Input: part model. Units: mm. Frame: model coordinates. Give positions to 0.01 mm unless a question says otherwise; leave off trailing zeros. Loops run counter-clockwise (first coordinate to the right, second up) from the corner with the lowest first, then second, coordinate; pieces in that order, holes last. Notation, with made-up numbers: (73.25, 84) -> (79.25, 84) arc R14 ccw to (79.25, 94) -> close; hole circle Ø1 at (39, 23.5). An arc over 180 degrees is marked (long way). Answer as a JSON object with one key per item and string values.
Autodesk Inventor part; units mm, degrees
ref_plane "YZ Plane" through (0, 0, 0) normal (1, 0, 0) x (0, 1, 0)
ref_plane "XZ Plane" through (0, 0, 0) normal (0, 1, 0) x (-1, 0, 0)
ref_plane "XY Plane" through (0, 0, 0) normal (0, 0, 1) x (1, 0, 0)
sketch "Sketch1" plane through (0, 0, 0) normal (0, 1, 0) x (-1, 0, 0)
  line L0 (1.9345, 2.6954) -> (3.3015, -0.3277)
  line L1 (3.3015, -0.3277) -> (1.367, -3.0231)
  line L2 (1.367, -3.0231) -> (-1.9345, -2.6954)
  line L3 (-1.9345, -2.6954) -> (-3.3015, 0.3277)
  line L4 (-3.3015, 0.3277) -> (-1.367, 3.0231)
  line L5 (-1.367, 3.0231) -> (1.9345, 2.6954)
  point P0 (0, 0)
  point P1 (0, 0)
extrude "Extrusion1" add sketch "Sketch1" along normal blind 19.05
sketch "Sketch2" plane through (0, 19.05, 0) normal (0, 1, 0) x (1, 0, 0)
  point P0 (0, 0)
  point P1 (0, 0)
hole "Hole1" at (0, 19.05, 0) direction (0, -1, 0) diameter 2.4892 end through all
properties part number "standoff"
Q1. Section C-C, the plane y = 2.5. Return the cut outline in (x, z).
Evaluation:
{"outline": "(-3.3, -0.33) -> (-1.37, -3.02) -> (1.93, -2.7) -> (3.3, 0.33) -> (1.37, 3.02) -> (-1.93, 2.7) -> close; hole circle Ø2.49 at (0, 0)"}
Q2. Ray query, line 1 along Z through (x, y) = (0, 5.25); line 2 along Z through (x, y) = (0.5, 10); line 3 along X through (y, z) = (5.25, 0). Return the intervals inside material, ascending.
Evaluation:
{"line 1": "z = -2.89 to -1.24, 1.24 to 2.89", "line 2": "z = -2.84 to -1.14, 1.14 to 2.94", "line 3": "x = -3.15 to -1.24, 1.24 to 3.15"}
Q3. Draft query along X for faces 1 (the cylindrical face through (-0.37, 9.39, 1.19)), 2 (the flat face through (0, 19.05, 1.4)), 3 (the flat face through (0.26, 9.39, -2.86)). Return one class per face: +X half, -X half, draft (parallel to the pull), parting line (faces both ways), or undercut.
Evaluation:
{"face 1": "undercut", "face 2": "draft", "face 3": "+X half"}
Q4. Section D-D, the plane z = -1.5. Return the cut outline in (x, y).
Evaluation:
{"outline": "(-2.46, 0) -> (2.48, 0) -> (2.48, 19.05) -> (-2.46, 19.05) -> close"}
Q5. Section A-A, the plane x = -0.75. Return the cut outline in (y, z).
Evaluation:
{"outline": "(0, -2.96) -> (19.05, -2.96) -> (19.05, -0.99) -> (0, -0.99) -> close; (0, 0.99) -> (19.05, 0.99) -> (19.05, 2.81) -> (0, 2.81) -> close"}
Q6. Pin query (flat end, axial travel): pin 1 (1 mm diameter, centred on x = -2.5, y = 7.5, fed in from -Z). Return the tip coordinate at first contact, or that it passes through.
Evaluation:
{"pin 1": "stops at z = -2.14"}
Q7. Section B-B, the plane z = -0.75. Return the cut outline in (x, y), then the cut area to 3 significant figures.
Evaluation:
{"outline": "(-3, 0) -> (-0.99, 0) -> (-0.99, 19.05) -> (-3, 19.05) -> close; (0.99, 0) -> (2.81, 0) -> (2.81, 19.05) -> (0.99, 19.05) -> close", "area": "72.9 mm2"}
